Verification items for this drawing (mm, ordinates from the low corner). A direction names the side the tool comes from. Give positions to 0.01 mm unless a question says otherwise; leave off trailing zeros. Write each loop counter-clockwise with the first axis right and the second up, starting at its lowest first coordinate (ties: lowest second). Pieces come first, ordered by that corner, then holes. Notation, with made-up numbers: (33, 59.5) -> (65, 59.5) arc R30 cw to (65, 97.5) -> close; hole circle Ø9 at (-14, -9). An arc over 180 degrees is marked (long way). Use one line per item in the form item = value. Start each with the question number.
(1) Section check C-C, the plane y = 2.5. Record the cut outline in (x, z) (3 decimals).
(2) Section check B-B, the plane x = 5.75. Record the cut outline in (y, z) (3 decimals).
(3) Section check A-A, the plane z = 12. Record the cut outline in (x, y), plus the area to 3 significant figures.
(4) Section check D-D, the plane x = 3.5. Record the cut outline in (y, z) (3 decimals), plus the area to 3 significant figures.
(5) Scan lines: L1, parallel to Y at x = 20.25, z = 12; L2, parallel to X at y = 11, z = 14.25; L3, parallel to Y at x = 4.75, z = 13.75. Record each from-to range of solid material in increasing order.
(6) Set-up check for the marked faces 1, 2 and 3: record each of +Z, -Z, +X, -X, +Y, -Y from which the full face is reachable in a straight line by a thin tool's end or side.
(7) Depth check by flat-ended pin: pin 1 Ø1.5 at (y, z) = (3, 11.5) entering from +X; pin 2 Ø1.5 at (x, y) = (6.5, 11) entering from +Z (3 decimals); pin 3 Ø4 at (x, z) = (6, 11) entering from -Y; pin 4 Ø2.5 at (x, y) = (5, 3.5) entering from -Z (3 decimals). Enter the tip coordinate at first touch or a pass-through.
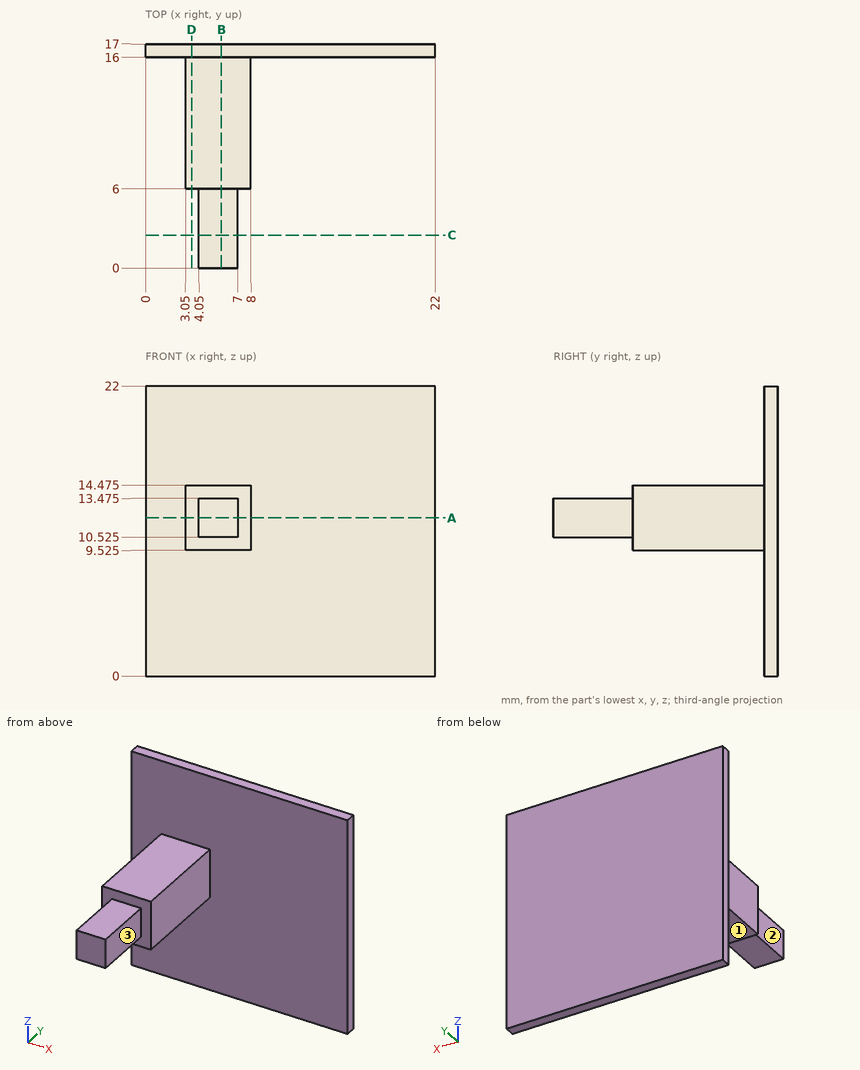
Completed:
q1.outline = (4.05, 10.525) -> (7, 10.525) -> (7, 13.475) -> (4.05, 13.475) -> close
q2.outline = (0, 10.525) -> (6, 10.525) -> (6, 9.525) -> (16, 9.525) -> (16, 0) -> (17, 0) -> (17, 22) -> (16, 22) -> (16, 14.475) -> (6, 14.475) -> (6, 13.475) -> (0, 13.475) -> close
q3.outline = (0, 16) -> (3.05, 16) -> (3.05, 6) -> (4.05, 6) -> (4.05, 0) -> (7, 0) -> (7, 6) -> (8, 6) -> (8, 16) -> (22, 16) -> (22, 17) -> (0, 17) -> close
q3.area = 89.2 mm²
q4.outline = (6, 9.525) -> (16, 9.525) -> (16, 0) -> (17, 0) -> (17, 22) -> (16, 22) -> (16, 14.475) -> (6, 14.475) -> close
q4.area = 71.5 mm²
q5.L1 = 16 to 17
q5.L2 = 3.05 to 8
q5.L3 = 6 to 17
q6.face_1 = -Z, +X, -X, -Y
q6.face_2 = +Z, -Z, -X, -Y
q6.face_3 = +Z, -Z, +X, -Y
q7.pin_1 = 7
q7.pin_2 = 14.475
q7.pin_3 = 0
q7.pin_4 = 10.525
